from build123d import *

# Parameters (mm, degrees)
SKETCH1_W           = 200
SKETCH1_H           = 10
BOSS_EXTRUDE1_DEPTH = 6
SKETCH2_W           = 54
SKETCH2_H           = 6.5
CUT_EXTRUDE1_DEPTH  = 15.5
FILLET1_R           = 6
FILLET2_R           = 5
CHAMFER1_SIZE       = 2
CUT_EXTRUDE2_DEPTH  = 31
SKETCH4_R           = 2.5
CUT_EXTRUDE3_DEPTH  = 31


# Some blends are built 0.0001 mm under size
with BuildPart() as part:
    # Sketch1 → Boss-Extrude1 (new, symmetric)
    with BuildSketch(Plane.XY):
        Rectangle(SKETCH1_W, SKETCH1_H)
    extrude(amount=BOSS_EXTRUDE1_DEPTH, both=True)

    # Sketch2 → Cut-Extrude1 (cut, symmetric)
    with BuildSketch(Plane(origin=(0, 0, 0), x_dir=(1, 0, 0), z_dir=(0, 1, 0))):
        with Locations((100, 6)):
            Rectangle(SKETCH2_W, SKETCH2_H)
        with Locations((100, -6)):
            Rectangle(SKETCH2_W, SKETCH2_H)
        with Locations((-100, -6)):
            Rectangle(SKETCH2_W, SKETCH2_H)
        with Locations((-100, 6)):
            Rectangle(SKETCH2_W, SKETCH2_H)
    extrude(amount=CUT_EXTRUDE1_DEPTH, both=True, mode=Mode.SUBTRACT)

    # Fillet1
    # the kernel refuses this fillet: 6 mm, written as the material it adds along each edge
    with BuildSketch(Plane(origin=(73, -5, -2.75), x_dir=(1, 0, 0), z_dir=(0, 1, 0)), Plane(origin=(-73, -5, 2.75), x_dir=(-1, 0, 0), z_dir=(0, 1, 0))) as fillet1_piece_1:
        with BuildLine():
            CenterArc((5.332682252, 6), FILLET1_R, 207.279612736, 62.720387264)
            Line((0, 3.25), (-0.106653645, 3.195))
            ThreePointArc((-0.106653645, 3.195), (-0.12, 1.625), (-0.12, 0))
            Line((-0.12, 0), (0, -0.12))
            Line((0, -0.12), (5.332682252, -0.12))
            Line((5.332682252, -0.12), (5.332682252, 0))
        make_face()
    extrude(amount=10)
    with BuildSketch(Plane(origin=(73, 5, 2.75), x_dir=(0, 0, 1), z_dir=(0, -1, 0)), Plane(origin=(-73, 5, -2.75), x_dir=(0, 0, -1), z_dir=(0, -1, 0))) as fillet1_piece_2:
        with BuildLine():
            CenterArc((6, -5.332682252), FILLET1_R, 117.279612736, 62.720387264)
            Line((0, -5.332682252), (-0.12, -5.332682252))
            Line((-0.12, -5.332682252), (-0.12, 0))
            Line((-0.12, 0), (0, 0.12))
            ThreePointArc((0, 0.12), (1.625, 0.12), (3.195, 0.106653645))
            Line((3.195, 0.106653645), (3.25, 0))
        make_face()
    extrude(amount=10)

    # Fillet2
    fillet2_edges = [part.edges().sort_by_distance(p)[0] for p in [
        (-100, -5, 0),
        (-100, 5, 0),
        (100, -5, 0),
        (100, 5, 0),
    ]]
    fillet(fillet2_edges, radius=FILLET2_R - 0.0001)  # a hair under: the kernel refuses the full size

    # Chamfer1
    chamfer1_edges = [part.edges().sort_by_distance(p)[0] for p in [
        (0, -5, -6),
        (0, 5, -6),
        (0, 5, 6),
        (0, -5, 6),
    ]]
    chamfer(chamfer1_edges, length=CHAMFER1_SIZE)

    # Sketch3 → Cut-Extrude2 (cut)
    with BuildSketch(Plane(origin=(0, 0, -6), x_dir=(-1, 0, 0), z_dir=(0, 0, -1))):
        with BuildLine():
            Line((-37.5, 1.75), (37.5, 1.75))
            ThreePointArc((37.5, 1.75), (39.25, 0), (37.5, -1.75))
            Line((37.5, -1.75), (-37.5, -1.75))
            ThreePointArc((-37.5, -1.75), (-39.25, 0), (-37.5, 1.75))
        make_face()
    extrude(amount=-CUT_EXTRUDE2_DEPTH, mode=Mode.SUBTRACT)

    # Sketch4 → Cut-Extrude3 (cut)
    with BuildSketch(Plane(origin=(0, 0, -2.75), x_dir=(-1, 0, 0), z_dir=(0, 0, -1))):
        with Locations((95, 0)):
            Circle(SKETCH4_R)
        with Locations((-95, 0)):
            Circle(SKETCH4_R)
    extrude(amount=-CUT_EXTRUDE3_DEPTH, mode=Mode.SUBTRACT)


solid = part.part
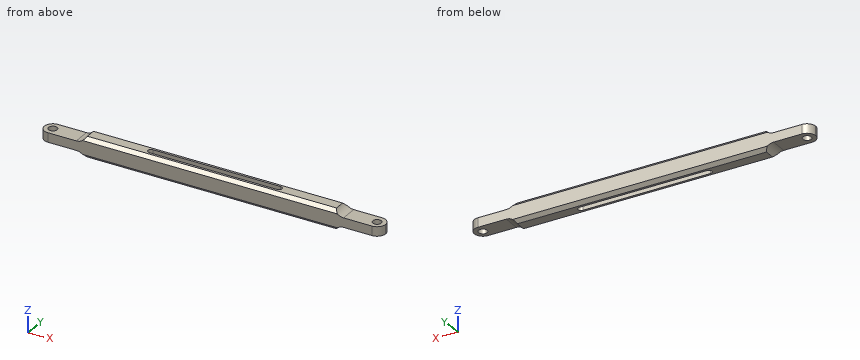
Can you work these out from the model? Positions are in its coordinate system, mm. Round coordinates to 2 decimals unless told otherwise and drop trailing zeros. Loops run counter-clockwise (first coordinate to the right, second up) from the corner with the lowest first, then second, coordinate; pieces in that order, holes last. Notation, with made-up numbers: (13.25, 87.5) - (55.25, 87.5) arc R18 cw to (55.25, 91.5) - close; hole circle Ø8 at (-20.5, -11.5). An arc over 180 degrees is marked (long way). Answer in a Markdown table with one row per item. Add a question column.
Q1. I want a section at B-B on z = -0.5. Count the separate pieces of the cut face and the enclosed holes in it, and give its area (3 significant figures).
Q2. I need wall thicknesses on L1, parallel to Y at x = 18.5, z = 2; L2, parallel to Y at x = 95, z = 1.15; L3, parallel to X at y = 2, z = -2.25. Which ranges of each line are inside material? Lowest first, please.
Q3. For pin 1 Ø6 at (y, z) = (-3.5, -1.5) entering from +X; pin 2 Ø5 at (x, y) = (94.5, 0) entering from +Z, each with a flat end and sliding along its axis, tell me the tip position at first contact or that it passes through.
Q4. I want a section at C-C on x = 57. List the corners of the cut face in (y, z) for me, and give its area (3 significant figures).
Q5. I want a section at A-A on x = 20.5. List the corners of the cut face in (y, z) for me.
A:
| question | item | result |
|---|---|---|
| 1 | separate pieces | 1 |
| 1 | enclosed holes | 3 |
| 1 | area | 1,670 mm^2 |
| 2 | L1 | -5 to -1.75, 1.75 to 5 |
| 2 | L2 | -5 to -2.5, 2.5 to 5 |
| 2 | L3 | -99.58 to -96.5, -93.5 to 93.5, 96.5 to 99.58 |
| 3 | pin 1 | x = 99.97 |
| 3 | pin 2 | z = 2.75 |
| 4 | outline | (-5, -4) - (-3, -6) - (3, -6) - (5, -4) - (5, 4) - (3, 6) - (-3, 6) - (-5, 4) - close |
| 4 | area | 112 mm^2 |
| 5 | outline | (-5, -4) - (-3, -6) - (-1.75, -6) - (-1.75, 6) - (-3, 6) - (-5, 4) - close; (1.75, -6) - (3, -6) - (5, -4) - (5, 4) - (3, 6) - (1.75, 6) - close |
